Input: part model. Units: mm. Frame: model coordinates. Face numbers are marked on the shaded views. A direction names the side the tool comes from. Round coordinates to 2 decimals unless told otherwise and drop trailing zeros. Write each loop counter-clockwise with the first axis right and the second up, starting at its lowest first coordinate (ties: lowest second). Pieces come first, ordered by that corner, then holes. Notation, with made-up numbers: (22.5, -16) - (33.5, -16) arc R20 ccw to (33.5, 13) - close; hole circle Ø2 at (62, 71.25). An arc over 180 degrees is marked (long way). One line per item, written item: value. Start each with the question number.
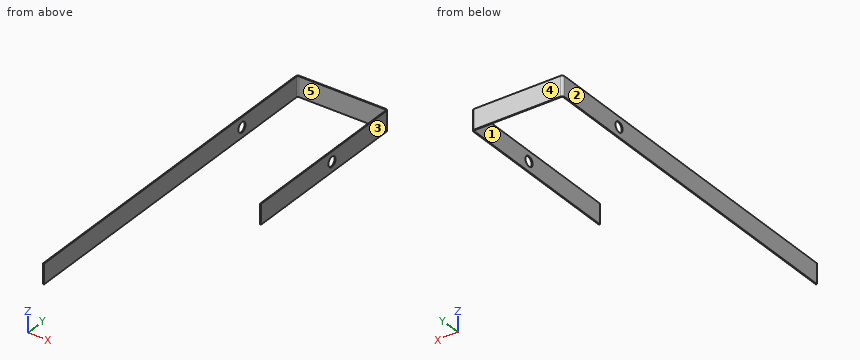
```python
from build123d import *

# Parameters (mm, degrees)
BASE_FLANGE3_DEPTH = 10
SKETCH15_R         = 2.5
CUT_EXTRUDE1_DEPTH = 45.72


# Sheet-metal steps are written as plain solids
with BuildPart() as part:
    # Sketch12 → Base-Flange3 (new body)
    with BuildSketch(Plane.XY):
        with BuildLine():
            Line((-70.950809652, -37.371859757), (-70.950809652, 139.183540243))
            ThreePointArc((-70.950809652, 139.183540243), (-70.586274752, 140.063605343), (-69.706209652, 140.428140243))
            Line((-69.706209652, 140.428140243), (-26.475409652, 140.428140243))
            ThreePointArc((-26.475409652, 140.428140243), (-25.595344552, 140.063605343), (-25.230809652, 139.183540243))
            Line((-25.230809652, 139.183540243), (-25.230809652, 51.528140243))
            Line((-25.230809652, 51.528140243), (-25.738809652, 51.528140243))
            Line((-25.738809652, 51.528140243), (-25.738809652, 139.183540243))
            ThreePointArc((-25.738809652, 139.183540243), (-25.954554797, 139.704395098), (-26.475409652, 139.920140243))
            Line((-26.475409652, 139.920140243), (-69.706209652, 139.920140243))
            ThreePointArc((-69.706209652, 139.920140243), (-70.227064507, 139.704395098), (-70.442809652, 139.183540243))
            Line((-70.442809652, 139.183540243), (-70.442809652, -37.371859757))
            Line((-70.442809652, -37.371859757), (-70.950809652, -37.371859757))
        make_face()
    extrude(amount=BASE_FLANGE3_DEPTH)

    # Sketch15 → Cut-Extrude1 (cut)
    with BuildSketch(Plane.ZY.offset(70.950809652)):
        with Locations((5, 101.083540243)):
            Circle(SKETCH15_R)
    extrude(amount=-CUT_EXTRUDE1_DEPTH, mode=Mode.SUBTRACT)


solid = part.part
```
Q1. Cut plane B-B, the plane y = 125. Output: boundary loops of the cut face in (x, z).
Q2. Pull-direction query (X, two-part tool) for the marked faces 3, 4 and 5; classes: pulls with the +X half, pulls with the -X half, needs draft (parallel to the pull), parting line crosses it, or undercut.
Q3. Cut plane D-D, the plane x = -61. Output: boundary loops of the cut face in (y, z), and give its area (3 significant figures).
Q4. Access query for the marked faces 1 and 2. Directions: +Z, -Z, +X, -X, +Y, -Y. A direction counts if a zero-diameter tool reaches every point of the face in a straight line with its end or side. Return the directions, or none.
Q5. Material intervals for probe 1 along X at (y, z) = (115, 7.5); probe 2 along Y at (x, z) = (-70.7, 5); probe 3 along Y at (x, z) = (-58, 4.75), sorted ascending. Write a range as from..to.
Q6. Cut plane C-C, the plane y = 49.5. Output: boundary loops of the cut face in (x, z), and give its area (3 significant figures).
Q7. Cut plane A-A, the plane z = 5. Output: boundary loops of the cut face in (x, y).
Q8. Contact query for a flat-ended pin moving along its axis: pin 1 Ø1 at (y, z) = (20, 6.5) entering from +X. Output: stop coordinate, or through.
A:
1. outline: (-70.95, 0) - (-70.44, 0) - (-70.44, 10) - (-70.95, 10) - close; (-25.74, 0) - (-25.23, 0) - (-25.23, 10) - (-25.74, 10) - close
2. face 3: pulls with the +X half
2. face 4: needs draft
2. face 5: undercut
3. outline: (139.92, 0) - (140.43, 0) - (140.43, 10) - (139.92, 10) - close
3. area: 5.08 mm²
4. face 1: +Z, -Z, -Y
4. face 2: +Z, -Z, -X, +Y, -Y
5. probe 1: x = -70.95..-70.44, -25.74..-25.23
5. probe 2: y = -37.37..98.58, 103.58..139.93
5. probe 3: y = 139.92..140.43
6. outline: (-70.95, 0) - (-70.44, 0) - (-70.44, 10) - (-70.95, 10) - close
6. area: 5.08 mm²
7. outline: (-70.95, -37.37) - (-70.44, -37.37) - (-70.44, 98.58) - (-70.95, 98.58) - close; (-70.95, 103.58) - (-70.44, 103.58) - (-70.44, 139.18) arc R0.74 cw to (-69.71, 139.92) - (-26.48, 139.92) arc R0.74 cw to (-25.74, 139.18) - (-25.74, 103.58) - (-25.23, 103.58) - (-25.23, 139.18) arc R1.24 ccw to (-26.48, 140.43) - (-69.71, 140.43) arc R1.24 ccw to (-70.95, 139.18) - close; (-25.74, 51.53) - (-25.23, 51.53) - (-25.23, 98.58) - (-25.74, 98.58) - close
8. pin 1: stops at x = -70.44
